For this review, take the finished solid that the model builds, in its own axes (mm). Face numbers are marked on the shaded views. A direction names the side the tool comes from. Give positions to 0.01 mm unless a question says otherwise; leave off trailing zeros. Write each loop counter-clockwise with the first axis right and the second up, starting at its lowest first coordinate (ties: lowest second). Pieces come first, ordered by that corner, then holes. Notation, with made-up numbers: M 78,19 L 127,19 A18 cw 127,37 Z; hole C 19,73.5 d5. An arc over 180 degrees is marked long. Write item = value, one per line.
```python
from build123d import *

# Parameters (mm, degrees)
SKETCH1_W           = 40
SKETCH1_H           = 40
SKETCH1_R           = 1.8
BOSS_EXTRUDE1_DEPTH = 7
SKETCH1_3_W         = 5
SKETCH1_3_H         = 40
BOSS_EXTRUDE2_DEPTH = 45
SKETCH2_R           = 1.8
CUT_EXTRUDE1_DEPTH  = 67.708320321
SKETCH2_4_OUTSIDE_W = 57.034
SKETCH2_4_OUTSIDE_H = 62.034
SKETCH2_4_OUTSIDE_R = 1.8
CUT_EXTRUDE2_DEPTH  = 67.708320321
FILLET1_R           = 5
FILLET2_R           = 5
FILLET3_R           = 1


with BuildPart() as part:
    # Sketch1 → Boss-Extrude1 (new body)
    with BuildSketch(Plane(origin=(0, 0, 0), x_dir=(1, 0, 0), z_dir=(0, 1, 0))):
        Rectangle(SKETCH1_W, SKETCH1_H)
        with Locations(Location((-5, -15, 0), (0, 0, 270))):
            Circle(SKETCH1_R, mode=Mode.SUBTRACT)
        with Locations(Location((15, -15, 0), (0, 0, 270))):
            Circle(SKETCH1_R, mode=Mode.SUBTRACT)
        with Locations(Location((-15, 15, 0), (0, 0, 270))):
            Circle(SKETCH1_R, mode=Mode.SUBTRACT)
        with Locations(Location((-5, 15, 0), (0, 0, 270))):
            Circle(SKETCH1_R, mode=Mode.SUBTRACT)
        with Locations(Location((5, 15, 0), (0, 0, 270))):
            Circle(SKETCH1_R, mode=Mode.SUBTRACT)
        with Locations(Location((15, 15, 0), (0, 0, 270))):
            Circle(SKETCH1_R, mode=Mode.SUBTRACT)
        with Locations(Location((5, -15, 0), (0, 0, 270))):
            Circle(SKETCH1_R, mode=Mode.SUBTRACT)
        with Locations(Location((-15, -15, 0), (0, 0, 270))):
            Circle(SKETCH1_R, mode=Mode.SUBTRACT)
    extrude(amount=BOSS_EXTRUDE1_DEPTH)

    # Sketch1<3> → Boss-Extrude2 (add)
    with BuildSketch(Plane(origin=(0, 0, 0), x_dir=(1, 0, 0), z_dir=(0, 1, 0))):
        with Locations((-22.5, 0)):
            Rectangle(SKETCH1_3_W, SKETCH1_3_H)
    extrude(amount=BOSS_EXTRUDE2_DEPTH)

    # Sketch2 → Cut-Extrude1 (cut, through all)
    with BuildSketch(Plane.ZY.offset(25)):
        with Locations((-15.5, 27.569)):
            Circle(SKETCH2_R)
        with BuildLine():
            Line((8, 20.569), (8, 34.569))
            ThreePointArc((8, 34.569), (0, 42.569), (-8, 34.569))
            Line((-8, 34.569), (-8, 20.569))
            ThreePointArc((-8, 20.569), (0, 12.569), (8, 20.569))
        make_face()
        with Locations((15.5, 27.569)):
            Circle(SKETCH2_R)
    extrude(amount=-CUT_EXTRUDE1_DEPTH, mode=Mode.SUBTRACT)

    # Sketch2<4> outside → Cut-Extrude2 (cut, through all)
    # profile 1 of 4: a face of its own
    with BuildSketch(Plane.ZY.offset(25)):
        with Locations((0, 22.5)):
            Rectangle(SKETCH2_4_OUTSIDE_W, SKETCH2_4_OUTSIDE_H)
        with BuildLine():
            Line((-20, 27.569), (-20, 0))
            Line((-20, 0), (20, 0))
            Line((20, 0), (20, 27.569))
            ThreePointArc((20, 27.569), (0, 47.569), (-20, 27.569))
        make_face(mode=Mode.SUBTRACT)
    # profile 2 of 4: a face of its own
    with BuildSketch(Plane.ZY.offset(25)):
        with Locations((-15.5, 27.569)):
            Circle(SKETCH2_4_OUTSIDE_R)
    # profile 3 of 4: a face of its own
    with BuildSketch(Plane.ZY.offset(25)):
        with Locations((15.5, 27.569)):
            Circle(SKETCH2_4_OUTSIDE_R)
    # profile 4 of 4: a face of its own
    with BuildSketch(Plane.ZY.offset(25)):
        with BuildLine():
            Line((-8, 20.569), (-8, 34.569))
            ThreePointArc((-8, 34.569), (0, 42.569), (8, 34.569))
            Line((8, 34.569), (8, 20.569))
            ThreePointArc((8, 20.569), (0, 12.569), (-8, 20.569))
        make_face()
    extrude(amount=-CUT_EXTRUDE2_DEPTH, mode=Mode.SUBTRACT)

    # Fillet1
    # the kernel refuses this fillet: 5 mm, written as the material it adds along each edge
    with BuildSketch(Plane(origin=(-20, 7, -20), x_dir=(1, 0, 0), z_dir=(0, 0, 1))) as fillet1_piece_1_section:
        with BuildLine():
            CenterArc((FILLET1_R, FILLET1_R), FILLET1_R, 180, 90)
            Line((0, FILLET1_R), (0, 0))
            Line((0, 0), (FILLET1_R, 0))
        make_face()
    fillet1_piece_1 = extrude(amount=40, mode=Mode.PRIVATE)
    fillet1_piece_1 = fillet1_piece_1 - Plane(origin=(-15, 8.140202128, -15), x_dir=(0, 0, 1), z_dir=(0, -1, 0)) * Cylinder(1.8, 100, mode=Mode.PRIVATE)
    fillet1_piece_1 = fillet1_piece_1 - Plane(origin=(-15, 8.140202128, 15), x_dir=(0, 0, 1), z_dir=(0, -1, 0)) * Cylinder(1.8, 100, mode=Mode.PRIVATE)
    add(fillet1_piece_1)

    # Fillet2
    # the kernel refuses this fillet: 5 mm, written as the material it takes off along each edge
    with BuildSketch(Plane(origin=(20, -12.5, -20), x_dir=(-1, 0, 0), z_dir=(0, 1, 0)), Plane(origin=(20, -12.5, 20), x_dir=(0, 0, -1), z_dir=(0, 1, 0))) as fillet2_piece_1:
        with BuildLine():
            CenterArc((FILLET2_R, FILLET2_R), FILLET2_R, 180, 90)
            Line((0, FILLET2_R), (0, 0))
            Line((0, 0), (FILLET2_R, 0))
        make_face()
    extrude(amount=32, mode=Mode.SUBTRACT)
    with BuildSketch(Plane(origin=(20, 7, 32.5), x_dir=(-1, 0, 0), z_dir=(0, 0, -1))) as fillet2_piece_2:
        with BuildLine():
            CenterArc((FILLET2_R, -FILLET2_R), FILLET2_R, 90, 90)
            Line((0, -FILLET2_R), (0, 0))
            Line((0, 0), (FILLET2_R, 0))
        make_face()
    extrude(amount=65, mode=Mode.SUBTRACT)

    # Fillet3
    fillet3_edges = [part.edges().sort_by_distance(p)[0] for p in [
        (-20, 37.665468331, -17.264452706),
        (-20, 37.665468331, 17.264452706),
        (0, 7, 20),
        (0, 7, -20),
        (-18.535533906, 8.464466094, -20),
        (-18.535533906, 8.464466094, 20),
        (18.816480084, 5.230244537, 18.230244537),
        (18.816480084, 5.230244537, -18.230244537),
        (-25, 45, 0),
        (-25, 13.7845, -20),
        (-20, 19.7845, -20),
        (-20, 19.7845, 20),
        (-25, 13.7845, 20),
        (-25, 37.665468331, -17.264452706),
        (-25, 37.665468331, 17.264452706),
    ]]
    fillet(fillet3_edges, radius=FILLET3_R)


solid = part.part
```
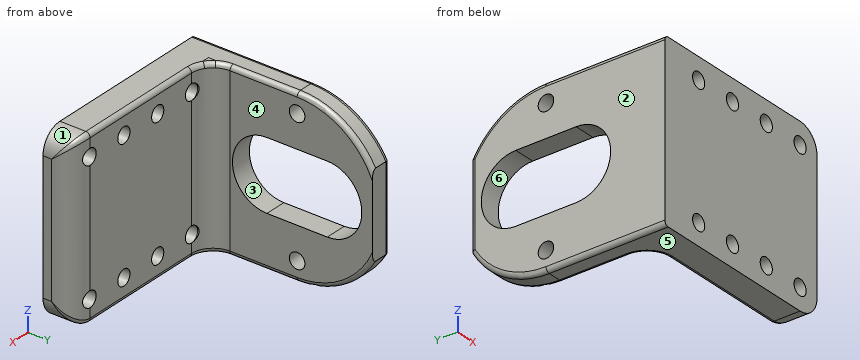
1. We need section A-A, the plane x = 5. Write out the cut boundary in (y, z), then the cut area to 3 significant figures.
Responses:
outline = M 0,-20 L 6,-20 A1 ccw 7,-19 L 7,-16.8 L 0,-16.8 Z; M 0,-13.2 L 7,-13.2 L 7,13.2 L 0,13.2 Z; M 0,16.8 L 7,16.8 L 7,19 A1 ccw 6,20 L 0,20 Z
area = 229 mm2
2. We need section B-B, the plane z = 0. Write out the cut boundary in (x, y).
Responses:
outline = M -25,0 L 20,0 L 20,2 A5 ccw 15,7 L -15,7 A5 cw -20,12 L -20,12.57 L -25,12.57 Z; M -25,42.57 L -20,42.57 L -20,45 L -24,45 A1 ccw -25,44 Z
3. For line 1 along X through (y, z) = (5, 15); line 2 along Z through (x, y) = (15, 2); line 3 along X through (y, z) = (1.75, -15), list the stretches that pass through material, from the lowest coordinate up. Write a range as from..to.
Responses:
line_1 = -25..-16.8, -13.2..-6.8, -3.2..3.2, 6.8..13.2, 16.8..19
line_2 = -20..-16.8, -13.2..13.2, 16.8..20
line_3 = -25..-16.8, -13.2..-6.8, -3.2..3.2, 6.8..13.2, 16.8..20
4. We need section C-C, the plane x = -8.5. Write out the cut boundary in (y, z), then the cut area to 3 significant figures.
Responses:
outline = M 0,-20 L 6,-20 A1 ccw 7,-19 L 7,19 A1 ccw 6,20 L 0,20 Z
area = 280 mm2
5. The part is to be moulded in two halves that separate along Z. For the marked faces 1, 2 and 3, say which applies: +Z half, -Z half, draft (parallel to the pull), parting line (faces both ways), or undercut.
Responses:
face_1 = +Z half
face_2 = draft
face_3 = undercut
6. Machinability: for the marked faces 4, 5 and 6, which of the approach directions +Z, -Z, +X, -X, +Y, -Y give a long, thin tool a straight path to every point of the face, cutting with its end or side? Answer none if there is none.
Responses:
face_4 = +Z, -Z, +X, +Y
face_5 = -Z, +X, -X, +Y, -Y
face_6 = +X, -X
7. Insertion check: P1, Ø3, axis at y = 27.569, z = -15.5, coming from the +X side; P2, Ø6, axis at x = -5, z = 15, coming from the +Y side; P3, Ø5, axis at x = -14.5, z = -4.5, coming from the +Y side; P4, Ø2.5, axis at x = -22.5, y = 30.5, coming from the +Z side. Each pin has a flat end and moves straight along its axis. Give the tip position at first contact, or say it passes through.
Responses:
P1 = through
P2 = 7
P3 = 7.42
P4 = 19.93
8. We need section D-D, the plane y = 5. Count the separate pieces of the cut face and the enclosed holes in it, then the cut area to 3 significant figures.
Responses:
separate_pieces = 1
enclosed_holes = 8
area = 1,670 mm2
